```python
from build123d import *

# Parameters (mm, degrees)
SKETCH_1_W          = 10
SKETCH_1_H          = 20
SKETCH_1_W_2        = 7
SKETCH_1_H_2        = 17
EXTRUDE_1_DEPTH     = 135
CUT_EXTRUDE_2_REACH = 138.839
SKETCH_3_R          = 2.15


with BuildPart() as part:
    # ｽｹｯﾁ1 → 押し出し-薄板1 (new body)
    with BuildSketch(Plane.XY):
        with Locations((5, 10)):
            Rectangle(SKETCH_1_W, SKETCH_1_H)
        with Locations((5, 10)):
            Rectangle(SKETCH_1_W_2, SKETCH_1_H_2, mode=Mode.SUBTRACT)
    extrude(amount=EXTRUDE_1_DEPTH)

    # ｶｯﾄ - 押し出し2: up to this face of the body (flat: up to its plane)
    cut_extrude_2_end = Plane(part.part.faces().sort_by_distance((0, 10, 67.5))[0])
    # ｽｹｯﾁ3 → ｶｯﾄ - 押し出し2 (cut, up to the picked face)
    with BuildSketch(Plane(origin=(10, 0, 0), x_dir=(0, 0, -1), z_dir=(1, 0, 0)), mode=Mode.PRIVATE) as cut_extrude_2_sk1:
        with Locations((-130, 15)):
            Circle(SKETCH_3_R)
    cut_extrude_2_tool1 = split(extrude(cut_extrude_2_sk1.sketch, amount=-CUT_EXTRUDE_2_REACH, mode=Mode.PRIVATE), bisect_by=cut_extrude_2_end, keep=Keep.BOTH, mode=Mode.PRIVATE)
    # ｽｹｯﾁ3 → ｶｯﾄ - 押し出し2 (cut, up to the picked face)
    with BuildSketch(Plane(origin=(10, 0, 0), x_dir=(0, 0, -1), z_dir=(1, 0, 0)), mode=Mode.PRIVATE) as cut_extrude_2_sk2:
        with Locations((-110, 15)):
            Circle(SKETCH_3_R)
    cut_extrude_2_tool2 = split(extrude(cut_extrude_2_sk2.sketch, amount=-CUT_EXTRUDE_2_REACH, mode=Mode.PRIVATE), bisect_by=cut_extrude_2_end, keep=Keep.BOTH, mode=Mode.PRIVATE)
    # ｽｹｯﾁ3 → ｶｯﾄ - 押し出し2 (cut, up to the picked face)
    with BuildSketch(Plane(origin=(10, 0, 0), x_dir=(0, 0, -1), z_dir=(1, 0, 0)), mode=Mode.PRIVATE) as cut_extrude_2_sk3:
        with Locations(Location((-25, 15, 0), (0, 0, 180))):
            Circle(SKETCH_3_R)
    cut_extrude_2_tool3 = split(extrude(cut_extrude_2_sk3.sketch, amount=-CUT_EXTRUDE_2_REACH, mode=Mode.PRIVATE), bisect_by=cut_extrude_2_end, keep=Keep.BOTH, mode=Mode.PRIVATE)
    # ｽｹｯﾁ3 → ｶｯﾄ - 押し出し2 (cut, up to the picked face)
    with BuildSketch(Plane(origin=(10, 0, 0), x_dir=(0, 0, -1), z_dir=(1, 0, 0)), mode=Mode.PRIVATE) as cut_extrude_2_sk4:
        with Locations(Location((-5, 15, 0), (0, 0, 180))):
            Circle(SKETCH_3_R)
    cut_extrude_2_tool4 = split(extrude(cut_extrude_2_sk4.sketch, amount=-CUT_EXTRUDE_2_REACH, mode=Mode.PRIVATE), bisect_by=cut_extrude_2_end, keep=Keep.BOTH, mode=Mode.PRIVATE)
    # ｽｹｯﾁ3 → ｶｯﾄ - 押し出し2 (cut, up to the picked face)
    with BuildSketch(Plane(origin=(10, 0, 0), x_dir=(0, 0, -1), z_dir=(1, 0, 0)), mode=Mode.PRIVATE) as cut_extrude_2_sk5:
        with Locations((-5, 5)):
            Circle(SKETCH_3_R)
    cut_extrude_2_tool5 = split(extrude(cut_extrude_2_sk5.sketch, amount=-CUT_EXTRUDE_2_REACH, mode=Mode.PRIVATE), bisect_by=cut_extrude_2_end, keep=Keep.BOTH, mode=Mode.PRIVATE)
    # ｽｹｯﾁ3 → ｶｯﾄ - 押し出し2 (cut, up to the picked face)
    with BuildSketch(Plane(origin=(10, 0, 0), x_dir=(0, 0, -1), z_dir=(1, 0, 0)), mode=Mode.PRIVATE) as cut_extrude_2_sk6:
        with Locations((-25, 5)):
            Circle(SKETCH_3_R)
    cut_extrude_2_tool6 = split(extrude(cut_extrude_2_sk6.sketch, amount=-CUT_EXTRUDE_2_REACH, mode=Mode.PRIVATE), bisect_by=cut_extrude_2_end, keep=Keep.BOTH, mode=Mode.PRIVATE)
    # ｽｹｯﾁ3 → ｶｯﾄ - 押し出し2 (cut, up to the picked face)
    with BuildSketch(Plane(origin=(10, 0, 0), x_dir=(0, 0, -1), z_dir=(1, 0, 0)), mode=Mode.PRIVATE) as cut_extrude_2_sk7:
        with Locations(Location((-110, 5, 0), (0, 0, 180))):
            Circle(SKETCH_3_R)
    cut_extrude_2_tool7 = split(extrude(cut_extrude_2_sk7.sketch, amount=-CUT_EXTRUDE_2_REACH, mode=Mode.PRIVATE), bisect_by=cut_extrude_2_end, keep=Keep.BOTH, mode=Mode.PRIVATE)
    # ｽｹｯﾁ3 → ｶｯﾄ - 押し出し2 (cut, up to the picked face)
    with BuildSketch(Plane(origin=(10, 0, 0), x_dir=(0, 0, -1), z_dir=(1, 0, 0)), mode=Mode.PRIVATE) as cut_extrude_2_sk8:
        with Locations(Location((-130, 5, 0), (0, 0, 180))):
            Circle(SKETCH_3_R)
    cut_extrude_2_tool8 = split(extrude(cut_extrude_2_sk8.sketch, amount=-CUT_EXTRUDE_2_REACH, mode=Mode.PRIVATE), bisect_by=cut_extrude_2_end, keep=Keep.BOTH, mode=Mode.PRIVATE)
    # ｽｹｯﾁ3 → ｶｯﾄ - 押し出し2 (cut, up to the picked face)
    with BuildSketch(Plane(origin=(10, 0, 0), x_dir=(0, 0, -1), z_dir=(1, 0, 0)), mode=Mode.PRIVATE) as cut_extrude_2_sk9:
        with Locations((-45, 10)):
            Circle(SKETCH_3_R)
    cut_extrude_2_tool9 = split(extrude(cut_extrude_2_sk9.sketch, amount=-CUT_EXTRUDE_2_REACH, mode=Mode.PRIVATE), bisect_by=cut_extrude_2_end, keep=Keep.BOTH, mode=Mode.PRIVATE)
    # ｽｹｯﾁ3 → ｶｯﾄ - 押し出し2 (cut, up to the picked face)
    with BuildSketch(Plane(origin=(10, 0, 0), x_dir=(0, 0, -1), z_dir=(1, 0, 0)), mode=Mode.PRIVATE) as cut_extrude_2_sk10:
        with Locations(Location((-90, 10, 0), (0, 0, 180))):
            Circle(SKETCH_3_R)
    cut_extrude_2_tool10 = split(extrude(cut_extrude_2_sk10.sketch, amount=-CUT_EXTRUDE_2_REACH, mode=Mode.PRIVATE), bisect_by=cut_extrude_2_end, keep=Keep.BOTH, mode=Mode.PRIVATE)
    add(cut_extrude_2_tool1.solids().sort_by(Axis((10, 15, 130), (-1, 0, 0)))[0], mode=Mode.SUBTRACT)
    add(cut_extrude_2_tool2.solids().sort_by(Axis((10, 15, 110), (-1, 0, 0)))[0], mode=Mode.SUBTRACT)
    add(cut_extrude_2_tool3.solids().sort_by(Axis((10, 15, 25), (-1, 0, 0)))[0], mode=Mode.SUBTRACT)
    add(cut_extrude_2_tool4.solids().sort_by(Axis((10, 15, 5), (-1, 0, 0)))[0], mode=Mode.SUBTRACT)
    add(cut_extrude_2_tool5.solids().sort_by(Axis((10, 5, 5), (-1, 0, 0)))[0], mode=Mode.SUBTRACT)
    add(cut_extrude_2_tool6.solids().sort_by(Axis((10, 5, 25), (-1, 0, 0)))[0], mode=Mode.SUBTRACT)
    add(cut_extrude_2_tool7.solids().sort_by(Axis((10, 5, 110), (-1, 0, 0)))[0], mode=Mode.SUBTRACT)
    add(cut_extrude_2_tool8.solids().sort_by(Axis((10, 5, 130), (-1, 0, 0)))[0], mode=Mode.SUBTRACT)
    add(cut_extrude_2_tool9.solids().sort_by(Axis((10, 10, 45), (-1, 0, 0)))[0], mode=Mode.SUBTRACT)
    add(cut_extrude_2_tool10.solids().sort_by(Axis((10, 10, 90), (-1, 0, 0)))[0], mode=Mode.SUBTRACT)


solid = part.part
```
Verification items for the finished model (mm, model axes). A direction names the side the tool comes from. Give positions to 0.01 mm unless a question says otherwise; leave off trailing zeros. Order: outer loops, then holes, each group sorted by start corner. A loop starts at its lowest first (then second) coordinate and runs counter-clockwise, first axis right, second up. Notation, with made-up numbers: M -8.5,-31.75 L 42.5,-31.75 A5 cw 42.5,-27.75 Z; hole C -19.75,2 d7. An arc over 180 degrees is marked long. Return JSON: item names as keys, results as strings. Group by question number.
1) Section check A-A on z = 90. Record the cut outline in (x, y).
2) Access from +Z, -Z, +X, -X, +Y, -Y to the whole of each face (thin tool, end or side, straight path). Record for faces 1 (the face through (8.5, 10, 67)), 2 (the face through (9.26, 17.1, 4.53)).
3) Go/stop test with a flat-tipped pin: pin 1 Ø1 at (x, y) = (3, 17.5) entering from -Z. Record where the tip stops, or that it passes through.
4) Section check C-C on y = 10. Record the cut outline in (x, z), and give its area (3 significant figures).
5) Mould release check, pull along X, two halves, no side actions. Record for faces 3 (the face through (5, 1.5, 67)), 4 (the face through (5, 20, 67)), 5 (the face through (0, 10, 67)): pulls with the +X half, pulls with the -X half, needs draft (parallel to the pull), parting line crosses it, or undercut.
6) Section check D-D on z = 57. Record the cut outline in (x, y).
7) Section check B-B on z = 130. Record the cut outline in (x, y).
8) Scan lines: line 1 (Y direction, x = 1.05, z = 25); line 2 (Y direction, x = 2.75, z = 14); line 3 (X direction, y = 17, z = 126). Record each from-to range of solid material in increasing order.
Answer block:
{
 "1": {"outline": "M 0,0 L 10,0 L 10,7.85 L 8.5,7.85 L 8.5,1.5 L 1.5,1.5 L 1.5,7.85 L 0,7.85 Z; M 0,12.15 L 1.5,12.15 L 1.5,18.5 L 8.5,18.5 L 8.5,12.15 L 10,12.15 L 10,20 L 0,20 Z"},
 "2": {"face 1": "+Z, -Z", "face 2": "+X, -X"},
 "3": {"pin 1": "passes through"},
 "4": {"outline": "M 0,0 L 1.5,0 L 1.5,42.85 L 0,42.85 Z; M 0,47.15 L 1.5,47.15 L 1.5,87.85 L 0,87.85 Z; M 0,92.15 L 1.5,92.15 L 1.5,135 L 0,135 Z; M 8.5,0 L 10,0 L 10,42.85 L 8.5,42.85 Z; M 8.5,47.15 L 10,47.15 L 10,87.85 L 8.5,87.85 Z; M 8.5,92.15 L 10,92.15 L 10,135 L 8.5,135 Z", "area": "379 mm^2"},
 "5": {"face 3": "undercut", "face 4": "needs draft", "face 5": "pulls with the -X half"},
 "6": {"outline": "M 0,0 L 10,0 L 10,20 L 0,20 Z; hole M 1.5,1.5 L 8.5,1.5 L 8.5,18.5 L 1.5,18.5 Z"},
 "7": {"outline": "M 0,0 L 10,0 L 10,2.85 L 8.5,2.85 L 8.5,1.5 L 1.5,1.5 L 1.5,2.85 L 0,2.85 Z; M 0,7.15 L 1.5,7.15 L 1.5,12.85 L 0,12.85 Z; M 0,17.15 L 1.5,17.15 L 1.5,18.5 L 8.5,18.5 L 8.5,17.15 L 10,17.15 L 10,20 L 0,20 Z; M 8.5,7.15 L 10,7.15 L 10,12.85 L 8.5,12.85 Z"},
 "8": {"line 1": "y = 0 to 2.85, 7.15 to 12.85, 17.15 to 20", "line 2": "y = 0 to 1.5, 18.5 to 20", "line 3": "x = 0 to 1.5, 8.5 to 10"}
}
